The model under review builds one solid part; all positions refer to its coordinate system, in mm. Face numbers are marked on the shaded views. A direction names the side the tool comes from. Coordinates: 2 decimals unless noted, no trailing zeros. Write each loop counter-clockwise with the first axis right and the second up, starting at its lowest first coordinate (ties: lowest second). Pieces come first, ordered by that corner, then holes. Notation, with made-up numbers: (-9, -7) - (5, -7) arc R10 ccw to (5, 8) - close; hole circle Ø9 at (58.5, 71.25). An arc over 180 degrees is marked (long way). Answer as CSV lines item,"result". Start each with the question number.
```python
from build123d import *

# Parameters (mm, degrees)
SKETCH_1_R      = 10
SKETCH_1_R_2    = 1.5
EXTRUDE_1_DEPTH = 2
SKETCH_2_R      = 3.203165256
SKETCH_2_R_2    = 2.072813242
EXTRUDE_2_DEPTH = 2.5


with BuildPart() as part:
    # 草图1 → 凸台-拉伸1 (new body)
    with BuildSketch(Plane(origin=(0, 0, 0), x_dir=(1, 0, 0), z_dir=(0, 1, 0))):
        with Locations(Location((0, 0, 0), (0, 0, 270))):
            Circle(SKETCH_1_R)
        with Locations(Location((0, 7, 0), (0, 0, 270))):
            Circle(SKETCH_1_R_2, mode=Mode.SUBTRACT)
        with Locations(Location((7, 0, 0), (0, 0, 270))):
            Circle(SKETCH_1_R_2, mode=Mode.SUBTRACT)
        with Locations(Location((0, -7, 0), (0, 0, 270))):
            Circle(SKETCH_1_R_2, mode=Mode.SUBTRACT)
        with Locations(Location((-7, 0, 0), (0, 0, 270))):
            Circle(SKETCH_1_R_2, mode=Mode.SUBTRACT)
        with Locations(Location((0, 0, 0), (0, 0, 270))):
            Circle(SKETCH_1_R_2, mode=Mode.SUBTRACT)
    extrude(amount=EXTRUDE_1_DEPTH)

    # 草图2 → 凸台-拉伸2 (add)
    with BuildSketch(Plane.XZ):
        with Locations(Location((0, 0, 0), (0, 0, 90))):
            Circle(SKETCH_2_R)
        with Locations(Location((0, 0, 0), (0, 0, 270))):
            Circle(SKETCH_2_R_2, mode=Mode.SUBTRACT)
    extrude(amount=EXTRUDE_2_DEPTH)


solid = part.part
```
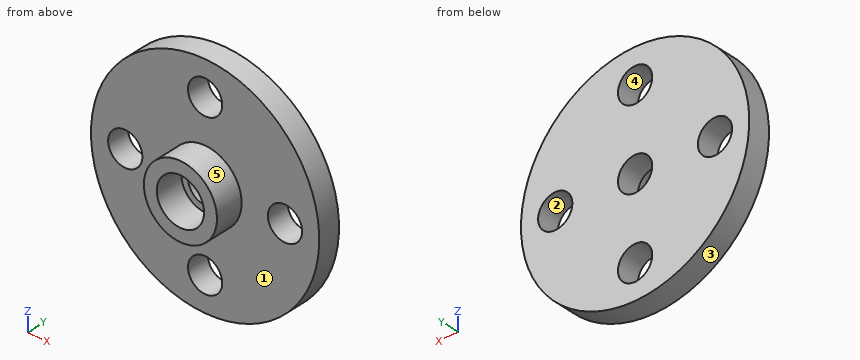
(1) For pin 1 (1 mm diameter, centred on x = -1, y = 0, fed in from -Z); pin 2 (3.5 mm diameter, centred on x = 0, z = 0, fed in from +Y); pin 3 (2 mm diameter, centred on x = 6, z = -1.5, fed in from -Y), all flat-tipped, find the tip position at first contact; note any pin that passes through.
(2) Wall thickness on line 1 (X direction, y = 0.6, z = 0); line 2 (X direction, y = 1.3, z = 1); line 3 (Y direction, x = -2, z = 4): over which ranges is each line inside the solid? List them lowest first.
(3) The part is to be moulded in two halves that separate along Z. For the marked faces 1, 2 and 3, say which applies: released by +Z, released by -Z, zero draft, split by the parting line, or undercut.
(4) Add section D-D on z = -7. Give the boundary of the cut face in (x, y).
(5) Add section B-B on x = 0. Give the boundary of the cut face in (y, z).
(6) For the marked faces 4 and 5, list the 3-axis set-ups (+Z, -Z, +X, -X, +Y, -Y) from which the entire face can be reached by the end or side of a thin tool; tool diameter is ignored.
(7) Add section A-A on z = 0. Give the boundary of the cut face in (x, y), then the cut area to 3 significant figures.
(8) Add section C-C on y = 0.95. Give the boundary of the cut face in (x, z), then the cut area to 3 significant figures.
Reported:
1,pin 1,"z = -9.99"
1,pin 2,"y = 2"
1,pin 3,"y = 0"
2,line 1,"-10 to -8.5, -5.5 to -1.5, 1.5 to 5.5, 8.5 to 10"
2,line 2,"-9.95 to -8.12, -5.88 to -1.12, 1.12 to 5.88, 8.12 to 9.95"
2,line 3,"0 to 2"
3,face 1,"zero draft"
3,face 2,"undercut"
3,face 3,"split by the parting line"
4,outline,"(-7.14, 0) - (-1.5, 0) - (-1.5, 2) - (-7.14, 2) - close; (1.5, 0) - (7.14, 0) - (7.14, 2) - (1.5, 2) - close"
5,outline,"(-2.5, -3.2) - (0, -3.2) - (0, -5.5) - (2, -5.5) - (2, -1.5) - (0, -1.5) - (0, -2.07) - (-2.5, -2.07) - close; (-2.5, 2.07) - (0, 2.07) - (0, 1.5) - (2, 1.5) - (2, 5.5) - (0, 5.5) - (0, 3.2) - (-2.5, 3.2) - close; (0, -10) - (2, -10) - (2, -8.5) - (0, -8.5) - close; (0, 8.5) - (2, 8.5) - (2, 10) - (0, 10) - close"
6,face 4,"+Y, -Y"
6,face 5,"-Y"
7,outline,"(-10, 0) - (-8.5, 0) - (-8.5, 2) - (-10, 2) - close; (-5.5, 0) - (-3.2, 0) - (-3.2, -2.5) - (-2.07, -2.5) - (-2.07, 0) - (-1.5, 0) - (-1.5, 2) - (-5.5, 2) - close; (1.5, 0) - (2.07, 0) - (2.07, -2.5) - (3.2, -2.5) - (3.2, 0) - (5.5, 0) - (5.5, 2) - (1.5, 2) - close; (8.5, 0) - (10, 0) - (10, 2) - (8.5, 2) - close"
7,area,"27.7 mm²"
8,outline,"circle Ø20 at (0, 0); hole circle Ø3 at (-7, 0); hole circle Ø3 at (0, -7); hole circle Ø3 at (0, 0); hole circle Ø3 at (0, 7); hole circle Ø3 at (7, 0)"
8,area,"279 mm²"
